Verification items for the finished model (mm, model axes). Face numbers are marked on the shaded views. A direction names the side the tool comes from. Coordinates: 2 decimals unless noted, no trailing zeros. Write each loop counter-clockwise with the first axis right and the second up, starting at its lowest first coordinate (ties: lowest second). Pieces come first, ordered by that corner, then holes. Notation, with made-up numbers: (49, -7.75) - (56, -7.75) arc R27 ccw to (56, 27.25) - close; hole circle Ø2 at (25, 17.25). An arc over 180 degrees is marked (long way). Use CSV: the item, a comma, the result in double quotes. Start each with the question number.
```python
from build123d import *

# Parameters (mm, degrees)
F1_DEPTH = 50
F3_DEPTH = 50.001
F5_DEPTH = 50


with BuildPart() as f1:
    # F0 (on Top) → F1 (new body)
    with BuildSketch(Plane.XY):
        Polygon((-49, 28.290163), (-49, -28.290163), (0, -56.580326), (49, -28.290163), (49, 28.290163), (0, 56.580326), align=None)
        Polygon((0, -51.961524), (-45, -25.980762), (-45, 25.980762), (0, 51.961524), (45, 25.980762), (45, -25.980762), align=None, mode=Mode.SUBTRACT)
    extrude(amount=F1_DEPTH)

    # F2 (on face) → F3 (cut, through all)
    with BuildSketch(Plane.XY.offset(50)):
        Polygon((0, 56.580326), (-49, 28.290163), (-47, 27.135463), (0, 54.270925), align=None)
        Polygon((49, -28.290163), (49, 28.290163), (47, 27.135463), (47, -27.135463), align=None)
        Polygon((-47, -27.135463), (-49, -28.290163), (0, -56.580326), (0, -54.270925), align=None)
    extrude(amount=-F3_DEPTH, mode=Mode.SUBTRACT)

    # F4 (on face) → F5 (join)
    with BuildSketch(Plane.XY.offset(50)):
        Polygon((-47, 27.135463), (-49, 28.290163), (-49, -28.290163), (-47, -27.135463), align=None)
        Polygon((49, 28.290163), (0, 56.580326), (0, 54.270925), (47, 27.135463), align=None)
        Polygon((0, -54.270925), (0, -56.580326), (49, -28.290163), (47, -27.135463), align=None)
    extrude(amount=F5_DEPTH)


solid = f1.part
```
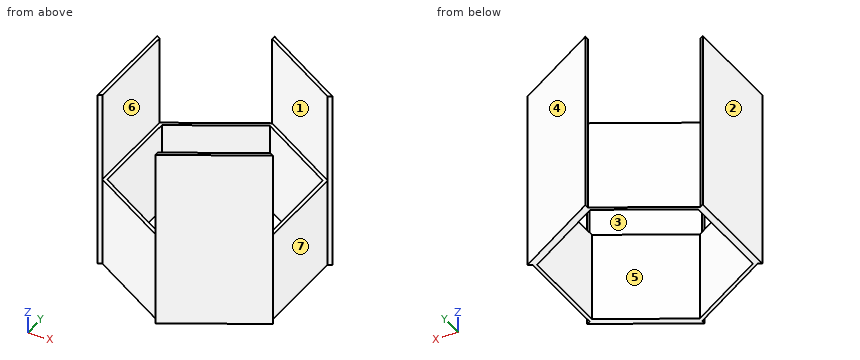
Q1. Tool access check on the marked faces 5, 6 and 7. Record the directions out of +Z, -Z, +X, -X, +Y, -Y that give a thin tool (end or side, any length) a straight path to the whole face; none if there is none.
Q2. Cross-section at D-D (z = 27.5). Record the cut outline in (x, y).
Q3. Cross-section at B-B (y = -18.5). Record the cut outline in (x, z).
Q4. Cross-section at C-C (x = 36). Record the cut outline in (y, z), plus the area to 3 significant figures.
Q5. Gauge pin test, flat ends, axial feed: pin 1 (2 mm diameter, centred on x = 21, z = 12.5, fed in from -Y); pin 2 (0.7 mm diameter, centred on y = 56, z = 44.5, fed in from -X); pin 3 (12 mm diameter, centred on y = -2.5, z = 12, fed in from +X). Record the tip position at first contact, or that the pin passes through.
Q6. Scan lines: line 1 along X through (y, z) = (-19, 28.5); line 2 along X through (y, z) = (28, 12); line 3 along Y through (x, z) = (-25, 38). Record each from-to range of solid material in increasing order. Write a range as from..to.
Q7. Cross-section at A-A (z = 76). Record the cut outline in (x, y), plus the area to 3 significant figures.
Q8. Release check for a two-part mould opening along Y. For the marked faces 1, 2, 3 and 4 record: released by +Y, released by -Y, zero draft, split by the parting line, or undercut.
Reply:
1,face 5,"+Z, -Z"
1,face 6,"+Z, +X, +Y, -Y"
1,face 7,"+Z, -Z, +X"
2,outline,"(-49, -28.29) - (-47, -27.14) - (0, -54.27) - (0, -56.58) - (49, -28.29) - (47, -27.14) - (47, 27.14) - (49, 28.29) - (0, 56.58) - (0, 54.27) - (-47, 27.14) - (-49, 28.29) - close; hole (-45, -25.98) - (0, -51.96) - (45, -25.98) - (45, 25.98) - (0, 51.96) - (-45, 25.98) - close"
3,outline,"(-49, 0) - (-45, 0) - (-45, 50) - (-47, 50) - (-47, 100) - (-49, 100) - close; (45, 0) - (47, 0) - (47, 50) - (45, 50) - close"
4,outline,"(-35.8, 0) - (-31.18, 0) - (-31.18, 50) - (-33.49, 50) - (-33.49, 100) - (-35.8, 100) - close; (31.18, 0) - (35.8, 0) - (35.8, 100) - (33.49, 100) - (33.49, 50) - (31.18, 50) - close"
4,area,"693 mm^2"
5,pin 1,"y = -45.03"
5,pin 2,"x = 0"
5,pin 3,"x = 47"
6,line 1,"-49..-45, 45..47"
6,line 2,"-49..-48.5, -45.5..-41.5, 41.5..48.5"
6,line 3,"-39.84..-37.53, 37.53..39.84"
7,outline,"(-49, -28.29) - (-47, -27.14) - (-47, 27.14) - (-49, 28.29) - close; (0, -56.58) - (49, -28.29) - (47, -27.14) - (0, -54.27) - close; (0, 54.27) - (47, 27.14) - (49, 28.29) - (0, 56.58) - close"
7,area,"333 mm^2"
8,face 1,"undercut"
8,face 2,"zero draft"
8,face 3,"undercut"
8,face 4,"released by +Y"
